Autodesk Fusion 360 part; units mm, degrees
sketch "Sketch1" plane through (0, 0, 0) normal (0, 1, 0) x (1, 0, 0)
  line L0 (25.4635, 63.881) -> (9.3726, 63.881)
  line L1 (9.3726, 63.881) -> (9.3726, 0)
  line L2 (9.3726, 0) -> (25.4635, 0)
  line L3 (25.4635, 0) -> (25.4635, 63.881)
  line L4 (15.7353, 0) -> (15.7353, 21.0056)
  line L5 (15.7353, 21.0056) -> (15.9893, 24.638)
  line L6 (15.9893, 24.638) -> (15.9893, 25.4)
  line L7 (15.9893, 25.4) -> (9.3726, 25.4)
  line L8 (0, 29.7705) -> (13.8983, 23.2896)
  dimension "d1" = 9.3726
  dimension "d2" = 25.4635
  dimension "d3" = 63.881
  dimension "d6" = 15.7353
  dimension "d7" = 0.762
  dimension "d8" = 4
  dimension "d9" = 25.4
  dimension "d10" = 0.254
  dimension "d11" = 65
revolve "Revolve1" add sketch "Sketch1" angle 360 about axis through (0, 0, 1.75) along (0, 0, 1) contours L0 L1 L2 L3 L4 L5 L6 L7
chamfer "Chamfer1" distance 0.762 angle 45 1 edges at (-23.7403, -9.208, 0)
equation "d1 = ( 0.738 / 2 ) * 1 in"
equation "d2 = 2.005 in / 2"
equation "d3 = 2.5 in + 0.015 in"
equation "d6 = ( 1.239 / 2 ) * 1 in"
equation "d11 = ( 130 / 2 ) * 1 deg"
CAD build for the part. Positions are in the model's coordinates, mm. A direction names the side the tool comes from. Round coordinates to 2 decimals unless told otherwise and drop trailing zeros. Write each loop counter-clockwise with the first axis right and the second up, starting at its lowest first coordinate (ties: lowest second). Pieces come first, ordered by that corner, then holes. Notation, with made-up numbers: M -14.75,-33.75 L 13.25,-33.75 A14 ccw 13.25,-6.75 Z; hole C 33.5,6 d6. An arc over 180 degrees is marked long. Use a Markdown table: item, result. Add a question column.
1. Pull direction Z, two halves, no side cores. Call faces 1 (the face through (-5.52, 24.86, -32.76)), 2 (the face through (15.05, -4.74, -21.64)), 3 (the face through (0, -11, -63.881)): released by +Z, released by -Z, zero draft, split by the parting line, or undercut.
2. Slice it at A-A on x = 0. Give the cut face in (y, z).
3. Slice it at D-D on z = -18.5. Give the cut face in (x, y).
4. Slice it at C-C on z = -31. Give the cut face in (x, y).
5. Drill centre lines: probe 1 along Y at (x, z) = (0, -38.5); probe 2 along X at (y, z) = (-8, -9); probe 3 along Y at (x, z) = (3, -44). Where is each one in solid material? Low to high.
6. Flat gauge pins, fed straight in: P1, Ø1.5, axis at x = -15, z = -8.5, coming from the +Y side; P2, Ø3, axis at x = -19, z = -53.5, coming from the -Y side; P3, Ø10, axis at y = 6.5, z = -25.5, coming from the -X side; P4, Ø17, axis at x = 0, y = 0, coming from the -Z side. Where does each tip first touch, or does it go through?
7. 3-axis set-ups, long thin cutter, end or side, ignore diameter. For faces 4 (the face through (8.459, -13.268, -10.65)), 5 (the face through (-12.69, 9.73, -25.02)), 6 (the face through (0, -16, 0)): which of +Z, -Z, +X, -X, +Y, -Y reach the whole face in a straight line?
Reply:
| question | item | result |
|---|---|---|
| 1 | face 1 | zero draft |
| 1 | face 2 | undercut |
| 1 | face 3 | released by -Z |
| 2 | outline | M -25.46,-63.88 L -9.37,-63.88 L -9.37,-25.4 L -15.99,-25.4 L -15.99,-24.64 L -15.74,-21.01 L -15.74,0 L -24.7,0 L -25.46,-0.76 Z; M 9.37,-63.88 L 25.46,-63.88 L 25.46,-0.76 L 24.7,0 L 15.74,0 L 15.74,-21.01 L 15.99,-24.64 L 15.99,-25.4 L 9.37,-25.4 Z |
| 3 | outline | C 0,0 d50.93; hole C 0,0 d31.47 |
| 4 | outline | C 0,0 d50.93; hole C 0,0 d18.75 |
| 5 | probe 1 | y = -25.46 to -9.37, 9.37 to 25.46 |
| 5 | probe 2 | x = -24.17 to -13.55, 13.55 to 24.17 |
| 5 | probe 3 | y = -25.29 to -8.88, 8.88 to 25.29 |
| 6 | P1 | stops at y = 21.1 |
| 6 | P2 | stops at y = -18.5 |
| 6 | P3 | stops at x = -25.42 |
| 6 | P4 | passes through |
| 7 | face 4 | +Z |
| 7 | face 5 | none |
| 7 | face 6 | +Z, +X, -X, +Y, -Y |
